Input: part model. Units: mm. Frame: model coordinates. Face numbers are marked on the shaded views. Coordinates: 2 decimals unless noted, no trailing zeros. Loops run counter-clockwise (first coordinate to the right, second up) from the corner with the lowest first, then second, coordinate; pieces in that order, holes last.
Item 1: Section C-C on z = -24. Return loops of the section in (x, y).
Item 2: Section A-A on y = 0. Return loops of the section in (x, z).
Item 3: Pull-direction query (X, two-part tool) for the marked faces 1, 2 and 3; classes: released by +X, released by -X, zero draft, split by the parting line, or undercut.
Item 4: Ray query, line 1 along Y through (x, z) = (0, -20); line 2 along Z through (x, y) = (9.75, 3.5); line 3 along X through (y, z) = (3, -22.5). Return the intervals inside material, ascending.
Item 5: Contact query for flat-ended pins moving along their axis: P1, Ø2, axis at x = -7.5, z = -27, coming from the +Y side; P2, Ø1.5, axis at x = 7, z = -26, coming from the +Y side; P3, Ø1.5, axis at y = 3.5, z = -11, coming from the +X side. Output: stop coordinate, or through.
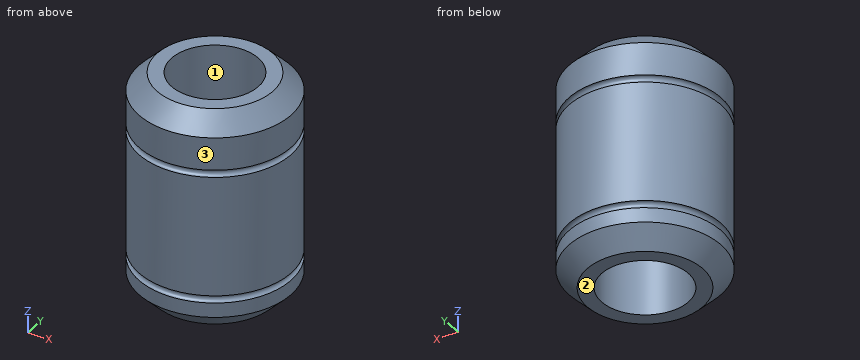
```python
from build123d import *

# Parameters (mm, degrees)
SKETCH_1_R      = 10.5
SKETCH_1_R_2    = 6
EXTRUDE_1_DEPTH = 30
SKETCH_4_R      = 0.5


with BuildPart() as part:
    # 草图1 → 凸台-拉伸1 (new body)
    with BuildSketch(Plane.XY):
        Circle(SKETCH_1_R)
        Circle(SKETCH_1_R_2, mode=Mode.SUBTRACT)
    extrude(amount=-EXTRUDE_1_DEPTH)

    # 草图2 → 切除-旋转3 (revolve, cut)
    with BuildSketch(Plane(origin=(0, 0, 0), x_dir=(1, 0, 0), z_dir=(0, 1, 0)), mode=Mode.PRIVATE) as cut_revolve_3_sk:
        Polygon((7.5, 30.5), (11, 27), (11, 30.5), align=None)
        Polygon((11, 3), (7.5, -0.5), (11, -0.5), align=None)
    revolve(cut_revolve_3_sk.sketch.rotate(Axis((0, 0, -40.551392487), (0, 0, 1)), 180), axis=Axis((0, 0, -40.551392487), (0, 0, 1)), mode=Mode.SUBTRACT)

    # 草图4 → 切除-旋转4 (revolve, cut)
    with BuildSketch(Plane(origin=(0, 0, 0), x_dir=(1, 0, 0), z_dir=(0, 1, 0)), mode=Mode.PRIVATE) as cut_revolve_4_sk:
        with Locations((10.5, 25)):
            Circle(SKETCH_4_R)
        with Locations((10.5, 7.5)):
            Circle(SKETCH_4_R)
    revolve(cut_revolve_4_sk.sketch.rotate(Axis((0, 0, -36.832356515), (0, 0, 1)), 180), axis=Axis((0, 0, -36.832356515), (0, 0, 1)), mode=Mode.SUBTRACT)


solid = part.part
```
Results found:
1. outline: circle Ø21 at (0, 0); hole circle Ø12 at (0, 0)
2. outline: (-10.5, -27.5) - (-8, -30) - (-6, -30) - (-6, 0) - (-8, 0) - (-10.5, -2.5) - (-10.5, -7) arc R0.5 cw to (-10.5, -8) - (-10.5, -24.5) arc R0.5 cw to (-10.5, -25.5) - close; (6, -30) - (8, -30) - (10.5, -27.5) - (10.5, -25.5) arc R0.5 cw to (10.5, -24.5) - (10.5, -8) arc R0.5 cw to (10.5, -7) - (10.5, -2.5) - (8, 0) - (6, 0) - close
3. face 1: undercut
3. face 2: zero draft
3. face 3: split by the parting line
4. line 1: y = -10.5 to -6, 6 to 10.5
4. line 2: z = -27.64 to -25.48, -24.52 to -7.98, -7.02 to -2.36
4. line 3: x = -10.06 to -5.2, 5.2 to 10.06
5. P1: stops at y = 8.25
5. P2: stops at y = 8.44
5. P3: stops at x = 10.13
